from build123d import *

# Parameters (mm, degrees)
SKETCH_1_W          = 13.5
SKETCH_1_H          = 6.2
EXTRUDE_1_DEPTH     = 16
SKETCH_2_W          = 3.25
SKETCH_2_H          = 1
EXTRUDE_2_DEPTH     = 6.2
SKETCH_3_R          = 0.75
CUT_EXTRUDE_1_DEPTH = 22.108410646
SKETCH_4_R          = 1.45
EXTRUDE_3_DEPTH     = 2.5
FILLET_1_SIZE       = 1
FILLET_1_SIZE_2     = 3
FILLET_2_SIZE       = 1
FILLET_2_SIZE_2     = 3
SKETCH_5_W          = 3
SKETCH_5_H          = 1
EXTRUDE_4_DEPTH     = 2


with BuildPart() as part:
    # 草图1 → 凸台-拉伸1 (new body)
    with BuildSketch(Plane(origin=(0, 0, 0), x_dir=(1, 0, 0), z_dir=(0, 1, 0))):
        with Locations((-6.75, 3.1)):
            Rectangle(SKETCH_1_W, SKETCH_1_H)
    extrude(amount=EXTRUDE_1_DEPTH)

    # 草图2 → 凸台-拉伸2 (add)
    with BuildSketch(Plane.XY):
        with Locations((1.625, 10.75)):
            Rectangle(SKETCH_2_W, SKETCH_2_H)
        with Locations((-15.125, 10.75)):
            Rectangle(SKETCH_2_W, SKETCH_2_H)
    extrude(amount=-EXTRUDE_2_DEPTH)

    # 草图3 → 切除-拉伸1 (cut, through all)
    with BuildSketch(Plane(origin=(0, 11.25, 0), x_dir=(1, 0, 0), z_dir=(0, 1, 0))):
        with Locations(Location((-15.25, 3.1, 0), (0, 0, 270))):
            Circle(SKETCH_3_R)
        with Locations(Location((1.75, 3.1, 0), (0, 0, 270))):
            Circle(SKETCH_3_R)
    extrude(amount=-CUT_EXTRUDE_1_DEPTH, mode=Mode.SUBTRACT)

    # 草图4 → 凸台-拉伸3 (add)
    with BuildSketch(Plane(origin=(0, 16, 0), x_dir=(1, 0, 0), z_dir=(0, 1, 0))):
        with Locations(Location((-10.35, 3.1, 0), (0, 0, 270))):
            Circle(SKETCH_4_R)
    extrude(amount=EXTRUDE_3_DEPTH)

    # 圆角1
    # an asymmetric fillet: 3, 1 mm, written as the material it takes off along each edge
    with BuildSketch(Plane(origin=(3.25, 2.75, 0), x_dir=(-1, 0, 0), z_dir=(0, 1, 0))) as fillet_1_piece_1:
        with BuildLine():
            Bezier((FILLET_1_SIZE, 0), (0, 0), (0, -FILLET_1_SIZE_2), weights=[1, 0.707106781, 1])
            Line((0, -FILLET_1_SIZE_2), (0, 0))
            Line((0, 0), (FILLET_1_SIZE, 0))
        make_face()
    extrude(amount=16, mode=Mode.SUBTRACT)
    with BuildSketch(Plane(origin=(-16.75, 2.75, -6.2), x_dir=(0, 0, 1), z_dir=(0, 1, 0))) as fillet_1_piece_2:
        with BuildLine():
            Bezier((FILLET_1_SIZE_2, 0), (0, 0), (0, FILLET_1_SIZE), weights=[1, 0.707106781, 1])
            Line((0, FILLET_1_SIZE), (0, 0))
            Line((0, 0), (FILLET_1_SIZE_2, 0))
        make_face()
    extrude(amount=16, mode=Mode.SUBTRACT)

    # 圆角2
    # an asymmetric fillet: 3, 1 mm, written as the material it takes off along each edge
    with BuildSketch(Plane(origin=(-16.75, 2.75, 0), x_dir=(1, 0, 0), z_dir=(0, 1, 0)), Plane(origin=(3.25, 2.75, -6.2), x_dir=(-1, 0, 0), z_dir=(0, 1, 0))) as fillet_2_piece_1:
        with BuildLine():
            Bezier((FILLET_2_SIZE, 0), (0, 0), (0, FILLET_2_SIZE_2), weights=[1, 0.707106781, 1])
            Line((0, FILLET_2_SIZE_2), (0, 0))
            Line((0, 0), (FILLET_2_SIZE, 0))
        make_face()
    extrude(amount=16, mode=Mode.SUBTRACT)

    # 草图5 → 凸台-拉伸4 (add)
    with BuildSketch(Plane.ZY.offset(13.5)):
        with Locations((-3.2, 0.5)):
            Rectangle(SKETCH_5_W, SKETCH_5_H)
    extrude(amount=EXTRUDE_4_DEPTH)


solid = part.part
The model under review builds one solid part; all positions refer to its coordinate system, in mm. A direction names the side the tool comes from. Give positions to 0.01 mm unless a question says otherwise; leave off trailing zeros. Write each loop counter-clockwise with the first axis right and the second up, starting at its lowest first coordinate (ties: lowest second). Pieces come first, ordered by that corner, then holes. Notation, with made-up numbers: M 44.25,35 L 96.25,35 A20 ccw 96.25,53 Z; hole C 56,0 d10. An arc over 180 degrees is marked long. One line per question, with ' | ' between items. Start each with the question number.
Item 1: Draft analysis for pull direction X (two halves, no side actions). For faces 5 (the flat face through (0, 14, -3)), 6 (the flat face through (-14.5, 0.5, -4.7)), 7 (the cylindrical face through (-14.74, 10.76, -3.65)), state which applies: released by +X, released by -X, zero draft, split by the parting line, or undercut.
Item 2: Wall thickness on line 1 (X direction, y = 10.85, z = -3.1); line 2 (Y direction, x = -14, z = -1.75); line 3 (Y direction, x = -4.5, z = -0.5): over which ranges is each line inside the solid? List them lowest first. Write a range as from..to.
Item 3: For faces 1 (the flat face through (1, 11.25, -2)), 2 (the flat face through (0, 5, -3)), 3 (the flat face through (-14, 1, -3)), 4 (the flat face through (-14, 11.25, -3)), list the 3-axis set-ups (+Z, -Z, +X, -X, +Y, -Y) from which the entire face can be reached by the end or side of a thin tool; tool diameter is ignored.
Item 4: We need section A-A on x = 1.75. Write out the cut boundary in (y, z).
Item 5: We need section D-D on x = -10.35. Write out the cut boundary in (y, z), plus the area to 3 significant figures.
Item 6: We need section B-B on x = -15.25. Write out the cut boundary in (y, z), plus the area to 3 significant figures.
Item 7: We need section C-C on y = 8.5. Write out the cut boundary in (x, z).
Item 8: For pin 1 (1.9 mm diameter, centred on y = 3.5, z = -4.5, fed in from +X); pin 2 (1.5 mm diameter, centred on y = 12.5, z = -4.5, fed in from -X); pin 3 (0.8 mm diameter, centred on y = 0.5, z = -3, fed in from -X), all flat-tipped, find the tip position at first contact; note any pin that passes through.
Results found:
1) face 5: released by +X | face 6: zero draft | face 7: undercut
2) line 1: x = -16.75..-16, -14.5..1, 2.5..3.25 | line 2: y = 0..1, 10.25..11.25 | line 3: y = 0..16
3) face 1: +Z, -Z, +X, +Y | face 2: +Z, -Z, +X, -Y | face 3: +Z, -Z, -X | face 4: +Z, -Z, -X, +Y
4) outline: M 10.25,-6.2 L 11.25,-6.2 L 11.25,-3.85 L 10.25,-3.85 Z; M 10.25,-2.35 L 11.25,-2.35 L 11.25,0 L 10.25,0 Z
5) outline: M 0,-6.2 L 16,-6.2 L 16,-4.55 L 18.5,-4.55 L 18.5,-1.65 L 16,-1.65 L 16,0 L 0,0 Z | area: 106 mm2
6) outline: M 0,-4.7 L 1,-4.7 L 1,-1.7 L 0,-1.7 Z; M 10.25,-6.2 L 11.25,-6.2 L 11.25,-3.85 L 10.25,-3.85 Z; M 10.25,-2.35 L 11.25,-2.35 L 11.25,0 L 10.25,0 Z | area: 7.70 mm2
7) outline: M -13.5,-6.2 L 0,-6.2 L 0,0 L -13.5,0 Z
8) pin 1: stops at x = 0 | pin 2: stops at x = -13.5 | pin 3: stops at x = -15.5
